from build123d import *

# Parameters (mm, degrees)
F1_DEPTH = 5
F3_DEPTH = 3


with BuildPart() as f1:
    # F0 (on Top) → F1 (new body)
    with BuildSketch(Plane.XY):
        with BuildLine():
            ThreePointArc((-95, -47), (-92.363961, -53.363961), (-86, -56))
            Line((-86, -56), (50, -56))
            Line((50, -56), (50, 56))
            Line((50, 56), (-86, 56))
            ThreePointArc((-86, 56), (-92.363961, 53.363961), (-95, 47))
            Line((-95, 47), (-95, -47))
        make_face()
    extrude(amount=F1_DEPTH)

    # F2 (on face) → F3 (cut)
    with BuildSketch(Plane.XY.offset(5)):
        with BuildLine():
            Line((50, -54), (50, 54))
            Line((50, 54), (-84, 54))
            ThreePointArc((-84, 54), (-90.363961, 51.363961), (-93, 45))
            Line((-93, 45), (-93, -45))
            ThreePointArc((-93, -45), (-90.363961, -51.363961), (-84, -54))
            Line((-84, -54), (50, -54))
        make_face()
    extrude(amount=-F3_DEPTH, mode=Mode.SUBTRACT)


solid = f1.part
Input: part model. Units: mm. Frame: model coordinates. A direction names the side the tool comes from. Round coordinates to 2 decimals unless told otherwise and drop trailing zeros. Loops run counter-clockwise (first coordinate to the right, second up) from the corner with the lowest first, then second, coordinate; pieces in that order, holes last. Notation, with made-up numbers: M 47.5,22 L 73.5,22 A23 ccw 73.5,31 Z; hole C 9.25,25.5 d3. An arc over 180 degrees is marked long. Answer as CSV lines item,"result". Start each with the question number.
(1) Draft query along Y for faces 3 (the flat face through (-19, -56, 2)), 4 (the flat face through (-93, 1, 4)), 5 (the flat face through (50, -1, 1)). Return one class per face: released by +Y, released by -Y, zero draft, split by the parting line, or undercut.
(2) Section C-C, the plane y = 22. Output: boundary loops of the cut face in (x, z), plus the area to 3 significant figures.
(3) Section A-A, the plane x = 25. Output: boundary loops of the cut face in (y, z), plus the area to 3 significant figures.
(4) First-contact query: pin 1 (8 mm diameter, centred on x = -45.5, y = 20, fed in from -Z); pin 2 (3 mm diameter, centred on y = -43.5, z = 4, fed in from +X). Flat tips, straight axial feed; report the tip coordinate or a pass-through.
(5) Line query: line 1 (Y direction, x = -82.5, z = 4.1); line 2 (X direction, y = -15.5, z = 4.4); line 3 (Z direction, x = 31.5, y = 17). Output: solid intervals per line, ascending. Write a range as [from, to].
(6) Section B-B, the plane z = 4.05. Output: boundary loops of the cut face in (x, y), plus the area to 3 significant figures.
(7) Reachability of faces 1 (the flat face through (-28.2, 54.2, 5)), 2 (the cylindrical face through (-90.434, -51.294, 3.521)) from +Z, -Z, +X, -X, +Y, -Y: full face, straight path, thin tool, end or side. Return the list, or none.
Values found:
1,face 3,"released by -Y"
1,face 4,"undercut"
1,face 5,"zero draft"
2,outline,"M -95,0 L 50,0 L 50,2 L -93,2 L -93,5 L -95,5 Z"
2,area,"296 mm²"
3,outline,"M -56,0 L 56,0 L 56,5 L 54,5 L 54,2 L -54,2 L -54,5 L -56,5 Z"
3,area,"236 mm²"
4,pin 1,"stops at z = 0"
4,pin 2,"stops at x = -93"
5,line 1,"y = [-56, -54], [54, 56]"
5,line 2,"x = [-95, -93]"
5,line 3,"z = [0, 2]"
6,outline,"M -95,-47 A9 ccw -86,-56 L 50,-56 L 50,-54 L -84,-54 A9 cw -93,-45 L -93,45 A9 cw -84,54 L 50,54 L 50,56 L -86,56 A9 ccw -95,47 Z"
6,area,"796 mm²"
7,face 1,"+Z, +X, -X, +Y, -Y"
7,face 2,"+Z, +X"
